Check sheet for the modelled part. Datum: model origin and axes. Units: mm. A direction names the side the tool comes from. Give positions to 0.01 mm unless a question says otherwise; leave off trailing zeros. Write each loop counter-clockwise with the first axis right and the second up, starting at its lowest first coordinate (ties: lowest second). Pieces come first, ordered by that corner, then holes. Notation, with made-up numbers: (-21, -14) -> (28, -14) arc R16 cw to (28, 8) -> close; hole circle Ø11 at (48, 2.25). An arc over 180 degrees is marked (long way). Use a Markdown table: item, result. Add a question column.
1. Release check for a two-part mould opening along X. For faces 4 (the flat face through (0, 28.575, 0)), 5 (the cylindrical face through (11.43, -26.13, -1.2)), 6 (the flat face through (28.575, 0, 0)), 7 (the flat face through (-28.575, 0, 0)) record: released by +X, released by -X, zero draft, split by the parting line, or undercut.
2. Set-up check for faces 1 (the cylindrical face through (17.9, -26.9, -3.7)), 2 (the cylindrical face through (27.04, 25.11, -0.14)), 3 (the cylindrical face through (-24.38, -13.83, 6.37)): record each of +Z, -Z, +X, -X, +Y, -Y from which the full face is reachable in a straight line by a thin tool's end or side.
3. Scan lines: probe 1 along X at (y, z) = (26.5, 5.5) (3 decimals); probe 2 along Y at (x, z) = (-23.5, 7.25) (3 decimals). Record each from-to range of solid material in increasing order. Write a range as [from, to].
4. Gauge pin test, flat ends, axial feed: P1, Ø2, axis at y = -12.7, z = 6.32, coming from the -X side; P2, Ø1.6, axis at x = 0, z = 0.03, coming from the -Y side; P3, Ø0.8, axis at y = 10, z = 2.5, coming from the +X side (3 decimals). Record the tip position at first contact, or that the pin passes through.
5. Cross-section at A-A (z = -3.25). Enter the section's corners in (x, y) (3 decimals).
from build123d import *

# Parameters (mm, degrees)
F0_W             = 57.15
F0_H             = 57.15
F1_DEPTH         = 10.12825
F2_R             = 2.1082
F3_DEPTH         = 3.429
F5_R             = 1.397
F6_DEPTH         = 20.2575
F8_D             = 2.2606
F8_DEPTH         = 8.2658857143
F8_TIP           = 0.6791527577
F9_R             = 1.27
F10_DEPTH        = 6.35
F12_D            = 2.2606
F12_DEPTH        = 8.255
F12_TIP          = 0.6791527577
F14_D            = 1.778
F14_DEPTH        = 4.826
F14_TIP          = 0.5341650903
F14_ON_F13_D     = 1.778
F14_ON_F13_DEPTH = 4.826
F14_ON_F13_TIP   = 0.5341650903


with BuildPart() as f1:
    # F0 (on Top) → F1 (new body, symmetric)
    with BuildSketch(Plane.XY):
        Rectangle(F0_W, F0_H)
    extrude(amount=F1_DEPTH, both=True)

    # F2 (on face) → F3 (cut)
    with BuildSketch(Plane.XZ.offset(28.575)):
        with Locations((-15.875, -4.28625)):
            Circle(F2_R)
        with Locations((15.875, -4.28625)):
            Circle(F2_R)
    extrude(amount=-F3_DEPTH, mode=Mode.SUBTRACT)

    # F5 (on face) → F6 (cut, through all)
    with BuildSketch(Plane(origin=(0, 0, -10.12825), x_dir=(1, 0, 0), z_dir=(0, 0, -1))):
        with Locations((-26.289, 26.289)):
            Circle(F5_R)
        with Locations((26.289, 26.289)):
            Circle(F5_R)
        with Locations((26.289, -26.289)):
            Circle(F5_R)
        with Locations((-26.289, -26.289)):
            Circle(F5_R)
    extrude(amount=-F6_DEPTH, mode=Mode.SUBTRACT)

    # F8
    with Locations(Plane(origin=(-28.575, 0, 0), x_dir=(0, -1, 0), z_dir=(-1, 0, 0))):
        with Locations((12.7, 6.31825), (-12.7, 6.31825)):
            Hole(F8_D / 2, depth=F8_DEPTH)
            with Locations((0, 0, -(F8_DEPTH + F8_TIP / 2))):  # 118° drill point
                Cone(0, F8_D / 2, F8_TIP, mode=Mode.SUBTRACT)

    # F9 (on face) → F10 (cut)
    with BuildSketch(Plane.YZ.offset(28.575)):
        with Locations((9.525, 2.00025)):
            Circle(F9_R)
    extrude(amount=-F10_DEPTH, mode=Mode.SUBTRACT)

    # F12
    with Locations(Plane.XZ.offset(28.575)):
        with Locations((-6.096, -7.08025), (0, -7.08025), (6.096, -7.08025)):
            Hole(F12_D / 2, depth=F12_DEPTH)
            with Locations((0, 0, -(F12_DEPTH + F12_TIP / 2))):  # 118° drill point
                Cone(0, F12_D / 2, F12_TIP, mode=Mode.SUBTRACT)

    # F14
    with Locations(Plane.XZ.offset(28.575)):
        with Locations((-21.209, -7.33425), (-10.541, -1.23825), (10.541, -1.23825), (21.209, -7.33425)):
            Hole(F14_D / 2, depth=F14_DEPTH)
            with Locations((0, 0, -(F14_DEPTH + F14_TIP / 2))):  # 118° drill point
                Cone(0, F14_D / 2, F14_TIP, mode=Mode.SUBTRACT)

    # F14 on F13
    with Locations(Plane.XZ.offset(28.575)):
        with Locations((0, 0.03175)):
            Hole(F14_ON_F13_D / 2, depth=F14_ON_F13_DEPTH)
            with Locations((0, 0, -(F14_ON_F13_DEPTH + F14_ON_F13_TIP / 2))):  # 118° drill point
                Cone(0, F14_ON_F13_D / 2, F14_ON_F13_TIP, mode=Mode.SUBTRACT)


solid = f1.part
Worked answers:
| question | item | result |
|---|---|---|
| 1 | face 4 | zero draft |
| 1 | face 5 | undercut |
| 1 | face 6 | released by +X |
| 1 | face 7 | released by -X |
| 2 | face 1 | -Y |
| 2 | face 2 | +Z, -Z |
| 2 | face 3 | -X |
| 3 | probe 1 | x = [-28.575, -27.67], [-24.908, 24.908], [27.67, 28.575] |
| 3 | probe 2 | y = [-28.575, -13.34], [-12.06, 12.06], [13.34, 28.575] |
| 4 | P1 | stops at x = -20.23 |
| 4 | P2 | stops at y = -23.7 |
| 4 | P3 | stops at x = 22.225 |
| 5 | outline | (-28.575, -28.575) -> (-17.711, -28.575) -> (-17.711, -25.146) -> (-14.039, -25.146) -> (-14.039, -28.575) -> (14.039, -28.575) -> (14.039, -25.146) -> (17.711, -25.146) -> (17.711, -28.575) -> (28.575, -28.575) -> (28.575, 28.575) -> (-28.575, 28.575) -> close; hole circle Ø2.794 at (-26.289, -26.289); hole circle Ø2.794 at (-26.289, 26.289); hole circle Ø2.794 at (26.289, -26.289); hole circle Ø2.794 at (26.289, 26.289) |
